```python
from build123d import *

# Parameters (mm, degrees)
SKETCH_1_R      = 2.5
EXTRUDE_1_DEPTH = 5
FILLET_2_R      = 11
FILLET_3_R      = 11


with BuildPart() as part:
    # 草图1 → 凸台-拉伸1 (new body)
    with BuildSketch(Plane(origin=(0, 0, 0), x_dir=(1, 0, 0), z_dir=(0, 1, 0))):
        with BuildLine():
            Line((11, -5), (-11, -5))
            ThreePointArc((-11, -5), (-16, 0), (-11, 5))
            Line((-11, 5), (11, 5))
            Line((11, 5), (117.253125833, 17.056349186))
            Line((117.253125833, 17.056349186), (120.081552958, 14.227922061))
            Line((120.081552958, 14.227922061), (132.809475019, 1.5))
            Line((132.809475019, 1.5), (132.809475019, -10.5))
            Line((132.809475019, -10.5), (127, -16))
            Line((127, -16), (119, -16))
            Line((119, -16), (19, -16))
            Line((19, -16), (11, -16))
            Line((11, -16), (11, -5))
        make_face()
        with Locations(Location((-11, 0, 0), (0, 0, 270))):
            Circle(SKETCH_1_R, mode=Mode.SUBTRACT)
        with Locations(Location((11, 0, 0), (0, 0, 270))):
            Circle(SKETCH_1_R, mode=Mode.SUBTRACT)
    extrude(amount=EXTRUDE_1_DEPTH)

    # 圆角2
    fillet_2_edges = [part.edges().sort_by_distance(p)[0] for p in [
        (11, 2.5, 5),
    ]]
    fillet(fillet_2_edges, radius=FILLET_2_R - 0.0001)  # a hair under: the kernel refuses the full size

    # 圆角3
    fillet_3_edges = [part.edges().sort_by_distance(p)[0] for p in [
        (11, 2.5, -5),
    ]]
    fillet(fillet_3_edges, radius=FILLET_3_R)


solid = part.part
```
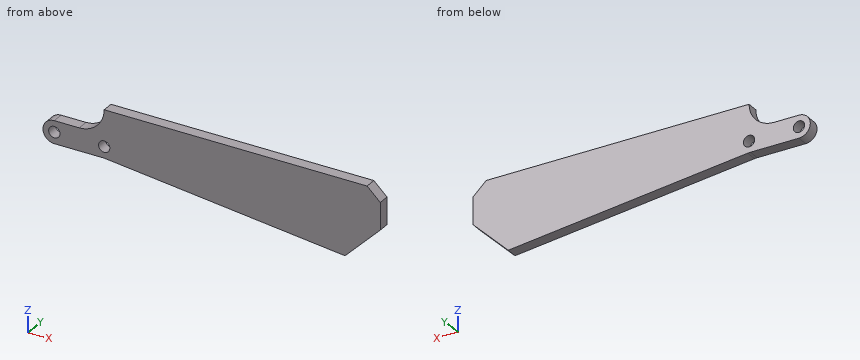
Build history of the part. All positions in model axes, mm. Coordinates: 2 decimals unless noted, no trailing zeros. Write each loop counter-clockwise with the first axis right and the second up, starting at its lowest first coordinate (ties: lowest second). Pieces come first, ordered by that corner, then holes.
1. Band-saw the part on C-C, the plane x = 74. Give the cut face in (y, z), and give its area (3 significant figures).
Answer block:
outline: (0, -12.15) - (5, -12.15) - (5, 16) - (0, 16) - close
area: 141 mm2
2. Drill centre lines: probe 1 along X at (y, z) = (2, 0); probe 2 along X at (y, z) = (1.15, -1); probe 3 along Z at (x, y) = (2.5, 1.45). Where is each one in solid material? Low to high.
Answer block:
probe 1: x = -16 to -13.5, -8.5 to 8.5, 13.5 to 132.81
probe 2: x = -15.9 to -13.29, -8.71 to 8.71, 13.29 to 132.81
probe 3: z = -5 to 5.29
3. Band-saw the part on A-A, the plane z = 0. Give the cut face in (x, y).
Answer block:
outline: (-16, 0) - (-13.5, 0) - (-13.5, 5) - (-16, 5) - close; (-8.5, 0) - (8.5, 0) - (8.5, 5) - (-8.5, 5) - close; (13.5, 0) - (132.81, 0) - (132.81, 5) - (13.5, 5) - close
4. Band-saw the part on D-D, the plane z = -13. Give the cut face in (x, y), and give its area (3 significant figures).
Answer block:
outline: (81.5, 0) - (121.31, 0) - (121.31, 5) - (81.5, 5) - close
area: 199 mm2
5. Band-saw the part on B-B, the plane y = 2.95. Give the number of separate pieces and of enclosed holes in the cut face, and give its area (3 significant figures).
Answer block:
separate pieces: 1
enclosed holes: 2
area: 3,500 mm2
6. Drop flat-ended pins along their axis: pin 1 (2 mm diameter, centred on x = 69, y = 3.5, fed in from -Z); pin 2 (1.5 mm diameter, centred on x = 0, y = 3, fed in from -Z). Give the stop position or say it passes through.
Answer block:
pin 1: stops at z = -11.69
pin 2: stops at z = -5
